Input: part model. Units: mm. Frame: model coordinates. Give positions to 0.01 mm unless a question says otherwise; leave off trailing zeros. Loops run counter-clockwise (first coordinate to the right, second up) from the corner with the lowest first, then second, coordinate; pieces in that order, holes last. Notation, with made-up numbers: M -13,-34 L 28,-34 A28 cw 28,-14 Z; hole C 73.5,10.5 d7. An arc over 180 degrees is marked long. Answer as a JSON object with one key per item and string values. Group by question number.
1) Section query A-A on z = 113. Return loops of the section in (x, y), plus the area to 3 significant figures.
2) Draft query along Z for faces 1 (the flat face through (74, 0, 887)), 2 (the flat face through (74, 353, 1202)), 3 (the flat face through (74, 592, 1800)). Return one class per face: +Z half, -Z half, draft (parallel to the pull), parting line (faces both ways), or undercut.
3) Ray query, L1, parallel to Y at x = 50, z = 479.5; L2, parallel to Y at x = 86, z = 1355.5; L3, parallel to Y at x = 100, z = 450.5. Return the intervals inside material, ascending.
4) Section query B-B on y = 77. Count the separate pieces of the cut face and the enclosed holes in it, plus the area to 3 significant figures.
from build123d import *

# Parameters (mm, degrees)
F0_W     = 1200
F0_H     = 1800
F1_DEPTH = 150
F2_W     = 1164
F2_H     = 1764
F3_DEPTH = 150
F4_W     = 150
F4_H     = 18
F5_DEPTH = 1764
F6_W     = 150
F6_H     = 18
F7_DEPTH = 660
F8_W     = 150
F8_H     = 18
F9_DEPTH = 486


with BuildPart() as f1:
    # F0 (on Right) → F1 (new body)
    with BuildSketch(Plane.YZ):
        with Locations((600, 900)):
            Rectangle(F0_W, F0_H)
    extrude(amount=F1_DEPTH)

    # F2 (on face) → F3 (cut)
    with BuildSketch(Plane.YZ.offset(150)):
        with Locations((600, 900)):
            Rectangle(F2_W, F2_H)
    extrude(amount=-F3_DEPTH, mode=Mode.SUBTRACT)

    # F4 (on face) → F5 (join)
    with BuildSketch(Plane.XY.offset(18)):
        with Locations((75, 687)):
            Rectangle(F4_W, F4_H)
    extrude(amount=F5_DEPTH)

    # F6 (on face) → F7 (join)
    with BuildSketch(Plane.XZ.offset(-678)):
        with Locations((75, 157)):
            Rectangle(F6_W, F6_H)
        with Locations((75, 305)):
            Rectangle(F6_W, F6_H)
        with Locations((75, 453)):
            Rectangle(F6_W, F6_H)
        with Locations((75, 601)):
            Rectangle(F6_W, F6_H)
        with Locations((75, 749)):
            Rectangle(F6_W, F6_H)
        with Locations((75, 897)):
            Rectangle(F6_W, F6_H)
        with Locations((75, 1045)):
            Rectangle(F6_W, F6_H)
        with Locations((75, 1193)):
            Rectangle(F6_W, F6_H)
        with Locations((75, 1341)):
            Rectangle(F6_W, F6_H)
        with Locations((75, 1489)):
            Rectangle(F6_W, F6_H)
    extrude(amount=F7_DEPTH)

    # F8 (on face) → F9 (join)
    with BuildSketch(Plane.XZ.offset(-1182)):
        with Locations((75, 177)):
            Rectangle(F8_W, F8_H)
        with Locations((75, 345)):
            Rectangle(F8_W, F8_H)
        with Locations((75, 513)):
            Rectangle(F8_W, F8_H)
        with Locations((75, 681)):
            Rectangle(F8_W, F8_H)
        with Locations((75, 849)):
            Rectangle(F8_W, F8_H)
        with Locations((75, 1017)):
            Rectangle(F8_W, F8_H)
        with Locations((75, 1185)):
            Rectangle(F8_W, F8_H)
        with Locations((75, 1353)):
            Rectangle(F8_W, F8_H)
        with Locations((75, 1521)):
            Rectangle(F8_W, F8_H)
    extrude(amount=F9_DEPTH)


solid = f1.part
Output:
{
 "1": {"outline": "M 0,0 L 150,0 L 150,18 L 0,18 Z; M 0,678 L 150,678 L 150,696 L 0,696 Z; M 0,1182 L 150,1182 L 150,1200 L 0,1200 Z", "area": "8,100 mm^2"},
 "2": {"face 1": "draft", "face 2": "undercut", "face 3": "+Z half"},
 "3": {"L1": "y = 0 to 18, 678 to 696, 1182 to 1200", "L2": "y = 0 to 18, 678 to 1200", "L3": "y = 0 to 696, 1182 to 1200"},
 "4": {"separate pieces": "12", "enclosed holes": "0", "area": "32,400 mm^2"}
}
